```python
from build123d import *

# Parameters (mm, degrees)
MODEL_W             = 57.154
MODEL_H             = 19.05137
MODEL_W_2           = 19.051
MODEL_H_2           = 19.051
MODEL_W_3           = 19.0514
MODEL_W_4           = 38.103
MODEL_W_5           = 38.1028
EXTRUDE_1_DEPTH     = 23.5
SKETCH_2_W          = 368.48
SKETCH_2_H          = 177.02
CUT_EXTRUDE_1_DEPTH = 16.5
CUT_EXTRUDE_2_DEPTH = 3


with BuildPart() as part:
    # Model → 凸台-拉伸1 (new body)
    with BuildSketch(Plane.XY):
        Polygon((-7.904930268, -7.726795577), (-7.935386074, 184.294), (375.473711158, 184.294), (375.566, -7.74368854), align=None)
        with Locations((160.494, 17.799415)):
            Rectangle(MODEL_W, MODEL_H, mode=Mode.SUBTRACT)
        Polygon((250.028, 142.579), (250.028, 123.963), (246.976, 138.322), (228.342, 134.36), (209.708, 130.4), (209.708, 130.401), (172.44, 122.479), (176.4, 103.845), (167.083, 101.865), (171.045, 83.228), (175.703, 84.2186), (179.663, 65.5863), (165.687, 62.6166), (169.649, 43.9801), (178.966, 45.9617), (182.926, 27.3279), (243.487, 40.2001), (243.487, 40.1987), (266.78, 45.1513), (258.859, 82.4205), (254.2, 81.431), (250.241, 100.062), (254.791, 101.03), (254.791, 82.568), (264.316, 82.568), (264.316, 63.518), (270.031, 63.518), (270.031, 44.468), (293.846, 44.468), (293.846, 63.518), (316.705, 63.518), (316.705, 82.568), (335.755, 82.568), (335.755, 101.621), (330.992, 101.621), (330.992, 120.671), (326.23, 120.671), (326.23, 139.721), (269.08, 139.721), (269.08, 142.579), align=None, mode=Mode.SUBTRACT)
        Polygon((79.6452, 120.831), (70.327, 122.811), (66.3663, 104.176), (71.0255, 103.185), (67.0648, 84.551), (76.382, 82.5722), (72.42, 63.9367), (72.4214, 63.9367), (68.4597, 45.303), (133.679, 31.4399), (133.679, 31.4413), (152.313, 27.4808), (156.275, 46.1162), (146.958, 48.0949), (150.919, 66.7286), (141.602, 68.7091), (145.562, 87.3428), (140.903, 88.3338), (144.865, 106.966), (154.182, 104.986), (158.142, 123.621), (139.507, 127.583), (139.507, 127.581), (83.6055, 139.464), align=None, mode=Mode.SUBTRACT)
        Polygon((321.466, 77.8083), (321.466, 58.7583), (302.416, 58.7583), (302.416, 39.7069), (359.569, 39.7069), (359.569, 58.7583), (340.517, 58.7583), (340.517, 77.8083), align=None, mode=Mode.SUBTRACT)
        Polygon((60.4795, 142.579), (60.4795, 139.721), (22.3807, 139.721), (22.3807, 120.671), (17.6182, 120.671), (17.6182, 101.621), (12.8557, 101.621), (12.8557, 82.5708), (8.09322, 82.5708), (8.09322, 44.468), (60.482, 44.468), (60.482, 63.518), (70.007, 63.518), (70.007, 82.5708), (65.2459, 82.5708), (65.2459, 120.671), (60.482, 120.671), (60.482, 123.526), (79.532, 123.526), (79.532, 142.579), align=None, mode=Mode.SUBTRACT)
        Polygon((326.227, 163.533), (326.227, 144.482), (330.991, 144.482), (330.991, 125.432), (335.753, 125.432), (335.753, 106.382), (340.516, 106.382), (340.516, 87.3319), (359.569, 87.3319), (359.569, 106.383), (354.806, 106.383), (354.806, 125.433), (350.042, 125.433), (350.042, 144.483), (345.28, 144.483), (345.28, 163.533), align=None, mode=Mode.SUBTRACT)
        Polygon((172.146, 146.761), (176.109, 128.126), (194.741, 132.086), (194.741, 132.085), (213.377, 136.047), (209.416, 154.682), align=None, mode=Mode.SUBTRACT)
        Polygon((117.205, 137.189), (154.474, 129.267), (158.434, 147.903), (121.165, 155.826), align=None, mode=Mode.SUBTRACT)
        Polygon((214.073, 155.673), (218.033, 137.036), (255.304, 144.959), (251.343, 163.594), align=None, mode=Mode.SUBTRACT)
        Polygon((75.2782, 146.101), (112.547, 138.18), (116.509, 156.815), (97.874, 160.776), (79.2399, 164.736), align=None, mode=Mode.SUBTRACT)
        with Locations((310.3225, 154.0075)):
            Rectangle(MODEL_W_2, MODEL_H_2, mode=Mode.SUBTRACT)
        with Locations((21.4292, 154.0075)):
            Rectangle(MODEL_W_3, MODEL_H_2, mode=Mode.SUBTRACT)
        with Locations((274.7945, 154.9595)):
            Rectangle(MODEL_W_4, MODEL_H_2, mode=Mode.SUBTRACT)
        with Locations((55.7195, 154.9595)):
            Rectangle(MODEL_W_5, MODEL_H_2, mode=Mode.SUBTRACT)
    extrude(amount=EXTRUDE_1_DEPTH)

    # 草图2 → 切除-拉伸1 (cut)
    with BuildSketch(Plane(origin=(0, 0, 0), x_dir=(-1, 0, 0), z_dir=(0, 0, -1))):
        with Locations((-183.826556737, 88.283426)):
            Rectangle(SKETCH_2_W, SKETCH_2_H)
    extrude(amount=-CUT_EXTRUDE_1_DEPTH, mode=Mode.SUBTRACT)

    # 草图3 → 切除-拉伸2 (cut)
    with BuildSketch(Plane(origin=(0, 0, 0), x_dir=(-1, 0, 0), z_dir=(0, 0, -1))):
        Polygon((-374.06527893, -6.243622428), (6.405168149, -6.226861644), (6.435148145, 182.794), (-373.97443185, 182.794), align=None)
    extrude(amount=-CUT_EXTRUDE_2_DEPTH, mode=Mode.SUBTRACT)


solid = part.part
```
Input: part model. Units: mm. Frame: model coordinates. A direction names the side the tool comes from. Coordinates: 2 decimals unless noted, no trailing zeros. Write each loop counter-clockwise with the first axis right and the second up, starting at its lowest first coordinate (ties: lowest second). Pieces come first, ordered by that corner, then holes. Notation, with made-up numbers: M 68.5,22 L 80.5,22 A16 ccw 80.5,30 Z; hole C -5.75,-30.75 d11. An arc over 180 degrees is marked long. Use one line per item in the form item = value.
Q1. Section C-C (x = 275). Return loops of the section in (y, z) (3 decimals).
Answer below:
outline = M -7.739,0 L -6.239,0 L -6.239,3 L -0.227,3 L -0.227,16.5 L 44.468,16.5 L 44.468,23.5 L -7.739,23.5 Z; M 139.721,16.5 L 145.434,16.5 L 145.434,23.5 L 139.721,23.5 Z; M 164.485,16.5 L 176.793,16.5 L 176.793,3 L 182.794,3 L 182.794,0 L 184.294,0 L 184.294,23.5 L 164.485,23.5 Z
Q2. Set-up query: faces 1 (the face through (186, 176.793, 10)), 2 (the face through (77.287, 155.549, 19.951)). Return all of +Z, -Z, +X, -X, +Y, -Y with unobstructed straight access to the full face (end or side cutting, diameter ignored); none if empty.
Answer below:
face_1 = -Z
face_2 = +Z, -Z
Q3. Section B-B (y = 115). Return loops of the section in (x, z).
Answer below:
outline = M -7.92,0 L -6.42,0 L -6.42,3 L -0.41,3 L -0.41,16.5 L 17.62,16.5 L 17.62,23.5 L -7.92,23.5 Z; M 65.25,16.5 L 68.67,16.5 L 68.67,23.5 L 65.25,23.5 Z; M 156.31,16.5 L 174.03,16.5 L 174.03,23.5 L 156.31,23.5 Z; M 330.99,16.5 L 335.75,16.5 L 335.75,23.5 L 330.99,23.5 Z; M 354.81,16.5 L 368.07,16.5 L 368.07,3 L 374.01,3 L 374.01,0 L 375.51,0 L 375.51,23.5 L 354.81,23.5 Z
Q4. Section D-D (y = 12). Return loops of the section in (x, z), plus the area to 3 significant figures.
Answer below:
outline = M -7.91,0 L -6.41,0 L -6.41,3 L -0.41,3 L -0.41,16.5 L 131.92,16.5 L 131.92,23.5 L -7.91,23.5 Z; M 189.07,16.5 L 368.07,16.5 L 368.07,3 L 374.06,3 L 374.06,0 L 375.56,0 L 375.56,23.5 L 189.07,23.5 Z
area = 2,500 mm²
Q5. Material intervals for probe 1 along X at (y, z) = (44.5, 2); probe 2 along Y at (x, z) = (162, 4.25); probe 3 along X at (y, z) = (70.5, 11.5), sorted ascending. Write a range as from..to.
Answer below:
probe_1 = -7.91..-6.41, 374.04..375.54
probe_2 = -7.73..-0.23, 176.79..184.29
probe_3 = -7.92..-0.41, 368.07..375.53
Q6. Section A-A (z = 10). Return loops of the section in (x, y).
Answer below:
outline = M -7.94,184.29 L -7.9,-7.73 L 375.57,-7.74 L 375.47,184.29 Z; hole M -0.41,-0.23 L 368.07,-0.23 L 368.07,176.79 L -0.41,176.79 Z
Q7. First-contact query: pin 1 (2 mm diameter, centred on x = 46.5, z = 20.5, fed in from -Y); pin 2 (7.5 mm diameter, centred on y = 71.5, z = 19, fed in from +X); pin 3 (3.5 mm diameter, centred on y = 76, z = 21, fed in from -X). Flat tips, straight axial feed; report the tip coordinate or a pass-through.
Answer below:
pin_1 = -7.73
pin_2 = 375.53
pin_3 = -7.92
